For this review, take the finished solid that the model builds, in its own axes (mm). Face numbers are marked on the shaded views. A direction names the side the tool comes from. Round coordinates to 2 decimals unless told otherwise and drop trailing zeros. Write each loop counter-clockwise with the first axis right and the second up, starting at its lowest first coordinate (ties: lowest second). Pieces come first, ordered by that corner, then holes. Notation, with made-up numbers: (-3.75, 46.25) -> (13.25, 46.25) arc R27 ccw to (13.25, 66.25) -> close; hole circle Ø5 at (83.5, 50.5). An arc over 180 degrees is marked (long way). Write item = value, one per line. Start each with the question number.
Autodesk Inventor part; units mm, degrees
ref_plane "YZ Plane" through (0, 0, 0) normal (1, 0, 0) x (0, 1, 0)
ref_plane "XZ Plane" through (0, 0, 0) normal (0, 1, 0) x (-1, 0, 0)
ref_plane "XY Plane" through (0, 0, 0) normal (0, 0, 1) x (1, 0, 0)
sketch "Sketch1" plane through (0, 0, 0) normal (0, 0, 1) x (1, 0, 0)
  line L0 (0, 0) -> (250, 0)
  line L1 (250, 0) -> (250, 250)
  line L2 (250, 250) -> (0, 250)
  line L3 (0, 250) -> (0, 0)
  dimension "d0" = 250
  dimension "d1" = 250
extrude "Extrusion1" add sketch "Sketch1" along normal blind 200
chamfer "Chamfer1" distance 100 distance2 40 1 edges at (0, 125, 0) measured on face at (0, 166.6667, 66.6667)
chamfer "Chamfer2" distance 100 distance2 40 1 edges at (145, 0, 0) measured on face at (180, 0, 66.6667)
chamfer "Chamfer3" distance 100 distance2 40 1 edges at (145, 250, 0) measured on face at (180, 250, 66.6667)
chamfer "Chamfer4" distance 100 distance2 40 1 edges at (250, 125, 0) measured on face at (250, 166.6667, 133.3333)
sketch "Sketch2" plane through (0, 0, 0) normal (0, 0, -1) x (-1, 0, 0)
  line L0 (-40, 40) -> (-210, 40)
  line L1 (-210, 210) -> (-40, 210)
  line L2 (-40, 40) -> (-210, 40)
  line L3 (-210, 40) -> (-210, 210)
  line L4 (-210, 210) -> (-40, 210)
  line L5 (-40, 210) -> (-40, 40)
  point P0 (0, 0)
extrude "Extrusion2" add sketch "Sketch2" along normal blind 150
sketch "Sketch3" plane through (40, 210, 0) normal (0, 1, 0) x (1, 0, 0)
  circle A0 centre (85, 110.8002) radius 20
  point P0 (-40, 0)
  dimension "d18" = 40
extrude "Extrusion3" add sketch "Sketch3" along normal blind 50
sketch "Sketch4" plane through (125, 260, -110.8002) normal (0, 1, 0) x (1, 0, 0)
  circle A0 centre (0, 0) radius 15
  point P0 (-125, -110.8002)
  dimension "d21" = 30
shell "Shell1" thickness 1 removed faces 1 at (83.3333, 166.6667, 200)
extrude "Extrusion4" cut sketch "Sketch4" against normal blind 60
sketch "Sketch5" plane through (40, 210, 0) normal (0, 1, 0) x (1, 0, 0)
  circle A0 centre (49.0593, 110.2763) radius 5
  point P0 (-40, 0)
  dimension "d25" = 10
extrude "Extrusion5" [suppressed]
sketch "Sketch6" plane through (89.0593, 290, -110.2763) normal (0, 1, 0) x (1, 0, 0)
  circle A0 centre (0, 0) radius 5
  line L0 (-5, 0) -> (5, 0)
  line L1 (5, 0) -> (5, -80.1533)
  line L2 (5, -80.1533) -> (-5, -80.1533)
  line L3 (-5, -80.1533) -> (-5, 0)
  point P0 (-89.0593, -110.2763)
extrude "Extrusion6" [suppressed]
sketch "Sketch7" plane through (0, 250, 100) normal (0, 0.9285, -0.3714) x (1, 0, 0)
  point P0 (0, 185.6953)
properties part number "my_subsystem"
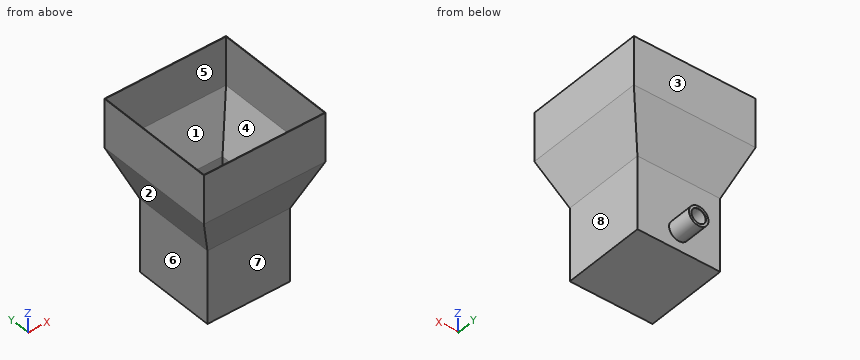
1. Consider section A-A, the plane x = 125. Give the boundary of the cut face in (y, z), then the cut area to 3 significant figures.
2. Clearance check with flat-ended pins moving along their axes: pin 1 Ø12 at (x, z) = (45.5, 122.5) entering from -Y; pin 2 Ø10 at (x, z) = (124.5, -24.5) entering from +Y; pin 3 Ø3 at (x, z) = (118.5, -89.5) entering from -Y; pin 4 Ø8 at (y, z) = (132.5, -108.5) entering from +X. State where each tip first meets the part, or that it passes through.
3. Wall thickness on L1, parallel to X at y = 230, z = 103.5; L2, parallel to Y at x = 66, z = -90: over which ranges is each line inside the solid? List them lowest first. Write a range as from..to.
4. Consider section C-C, the plane y = 233. Give the boundary of the cut face in (x, z).
5. Consider section D-D, the plane x = 190. Give the boundary of the cut face in (y, z), then the cut area to 3 significant figures.
6. Draft analysis for pull direction Y (two halves, no side actions). For the marked faces 1, 2, 3 and 4, state which applies: +Y half, -Y half, draft (parallel to the pull), parting line (faces both ways), or undercut.
7. Consider section B-B, the plane z = -55. Give the boundary of the cut face in (x, y), then the cut area to 3 significant figures.
8. Machinability: for the marked faces 5, 6, 7 and 8, which of the approach directions +Z, -Z, +X, -X, +Y, -Y give a long, thin tool a straight path to every point of the face, cutting with its end or side? Answer none if there is none.
Outcome:
q1.outline = (0, 100) -> (40, 0) -> (40, -150) -> (210, -150) -> (210, -130.8) -> (260, -130.8) -> (260, -125.8) -> (259, -125.8) -> (259, -129.8) -> (209, -129.8) -> (209, -149) -> (41, -149) -> (41, 0.19) -> (1, 100.19) -> (1, 200) -> (0, 200) -> close; (209, -91.8) -> (259, -91.8) -> (259, -95.8) -> (260, -95.8) -> (260, -90.8) -> (210, -90.8) -> (210, 0) -> (250, 100) -> (250, 200) -> (249, 200) -> (249, 100.19) -> (209, 0.19) -> close
q1.area = 953 mm2
q2.pin_1 = 0
q2.pin_2 = 210
q2.pin_3 = 40
q2.pin_4 = 210
q3.L1 = 0..1, 249..250
q3.L2 = 40..41, 209..210
q4.outline = (0, 100) -> (17, 57.5) -> (233, 57.5) -> (250, 100) -> (250, 200) -> (249, 200) -> (249, 100.19) -> (233, 60.19) -> (17, 60.19) -> (1, 100.19) -> (1, 200) -> (0, 200) -> close; circle Ø40 at (125, -110.8); hole circle Ø38 at (125, -110.8)
q5.outline = (0, 100) -> (40, 0) -> (40, -150) -> (210, -150) -> (210, 0) -> (250, 100) -> (250, 200) -> (249, 200) -> (249, 100.19) -> (209, 0.19) -> (209, -149) -> (41, -149) -> (41, 0.19) -> (1, 100.19) -> (1, 200) -> (0, 200) -> close
q5.area = 883 mm2
q6.face_1 = undercut
q6.face_2 = draft
q6.face_3 = +Y half
q6.face_4 = undercut
q7.outline = (40, 40) -> (210, 40) -> (210, 210) -> (40, 210) -> close; hole (41, 41) -> (209, 41) -> (209, 209) -> (41, 209) -> close
q7.area = 676 mm2
q8.face_5 = +Z
q8.face_6 = -Z, -X, +Y, -Y
q8.face_7 = -Z, +X, -X, -Y
q8.face_8 = -Z, +X, +Y, -Y
